Can you work these out from the model? Positions are in its coordinate system, mm. A direction names the side the tool comes from. Give positions to 0.01 mm unless a question says otherwise; leave off trailing zeros. Write each loop counter-clockwise with the first axis right and the second up, starting at its lowest first coordinate (ties: lowest second). Pieces come first, ordered by that corner, then holes.
1. If I drill on probe 1 along X at (y, z) = (21, 17); probe 2 along Y at (x, z) = (34, 2); probe 3 along X at (y, z) = (36, 21), over which ranges is the centre line in solid material (lowest first)?
2. Suppose I cut it at D-D (y = 75). Please give me the cut outline in (x, z), and give its area (3 significant figures).
3. Suppose I cut it at A-A (y = 36.5). Please give me the cut outline in (x, z), and give its area (3 significant figures).
4. Thinking about a two-plate mould opening in Y: for faces 5 (the flat face through (0, -20, 33.02)), 6 (the flat face through (-42.45, -34.32, 12.52)), 7 (the cylindrical face through (16.94, -31.6, 12.88)), which applies, pulls with the +Y half, pulls with the -Y half, needs draft (parallel to the pull), parting line crosses it, or undercut?
5. Suppose I cut it at C-C (z = 18). Please give me the cut outline in (x, y), and give its area (3 significant figures).
6. On a 3-axis mill with a long thin cutter (end or side, diameter ignored), from which of +Z, -Z, +X, -X, +Y, -Y can I reach the whole of each face in a straight line? I mean faces 1 (the flat face through (5.662, 2, 28)), 2 (the cylindrical face through (4.13, -25.59, 27.98)), 3 (the cylindrical face through (4.13, 31.13, 27.98)), 4 (the cylindrical face through (1.708, 21.837, 31.732)). Say none if no direction works.
7. Suppose I cut it at B-B (x = -54.5). Please give me the cut outline in (y, z).
8. I'm going to push flat-ended pins straight in: pin 1 (6 mm diameter, centred on x = 0, y = -11, fed in from +Z); pin 2 (1.1 mm diameter, centred on x = 0, z = 27, fed in from +Y); pin 3 (4 mm diameter, centred on y = 71.5, z = 5, fed in from -X). Where does each tip first touch, or does it pass through?
```python
from build123d import *

# Parameters (mm, degrees)
F1_DEPTH = 25.4
F2_R     = 10.16
F3_R     = 14.427985
F4_DEPTH = 25.401
F6_DEPTH = 5.08
F7_R     = 3.702221
F7_R_2   = 3.8131
F8_DEPTH = 2.54
F9_R     = 5.08


with BuildPart() as f1:
    # F0 (on Top) → F1 (new body)
    with BuildSketch(Plane.XY):
        with BuildLine():
            Line((-0.25744, -76.898574), (75.94256, 0))
            ThreePointArc((75.94256, 0), (-0.25744, 87.97693), (-76.45744, 0))
            Line((-76.45744, 0), (-0.25744, -76.898574))
        make_face()
    extrude(amount=F1_DEPTH)

    # F2
    f2_edges = [f1.edges().sort_by_distance(p)[0] for p in [
        (-0.25744, -76.898574, 12.7),
    ]]
    fillet(f2_edges, radius=F2_R)

    # F3 (on face) → F4 (cut, through all)
    with BuildSketch(Plane.XY.offset(25.4)):
        with Locations((0, 64.553022)):
            Circle(F3_R)
        with Locations((-45.933198, 31.180601)):
            Circle(F3_R)
        with Locations((-28.388277, -22.817112)):
            Circle(F3_R)
        with Locations((28.388277, -22.817112)):
            Circle(F3_R)
        with Locations((45.933198, 31.180601)):
            Circle(F3_R)
    extrude(amount=-F4_DEPTH, mode=Mode.SUBTRACT)

    # F5 (on face) → F6 (join)
    with BuildSketch(Plane.XY.offset(25.4)):
        Polygon((5.661786, 32.575481), (-6.728922, 32.575481), (-5.72427, -27.033882), (5.661786, -27.033882), align=None)
    extrude(amount=F6_DEPTH)

    # F7 (on face) → F8 (join)
    with BuildSketch(Plane.XY.offset(30.48)):
        with Locations((0, 25.121083)):
            Circle(F7_R)
        with Locations((0, -19.945145)):
            Circle(F7_R_2)
    extrude(amount=F8_DEPTH)

    # F9
    f9_edges = [f1.edges().sort_by_distance(p)[0] for p in [
        (-5.72427, -27.033882, 27.94),
        (5.661786, -27.033882, 27.94),
        (5.661786, 32.575481, 27.94),
        (-6.728922, 32.575481, 27.94),
    ]]
    fillet(f9_edges, radius=F9_R)


solid = f1.part
```
Checks:
1. probe 1: x = -76.59 to -56.16, -35.71 to 35.71, 56.16 to 76.08
1. probe 2: y = -42.33 to -36.11, -9.53 to 23.07, 39.29 to 79.94
1. probe 3: x = -73.07 to -59.53, -32.33 to 32.33, 59.53 to 72.55
2. outline: (-43.03, 0) - (-9.95, 0) - (-9.95, 25.4) - (-43.03, 25.4) - close; (9.95, 0) - (42.52, 0) - (42.52, 25.4) - (9.95, 25.4) - close
2. area: 1,670 mm2
3. outline: (-72.9, 0) - (-59.34, 0) - (-59.34, 25.4) - (-72.9, 25.4) - close; (-32.52, 0) - (32.52, 0) - (32.52, 25.4) - (-32.52, 25.4) - close; (59.34, 0) - (72.38, 0) - (72.38, 25.4) - (59.34, 25.4) - close
3. area: 2,330 mm2
4. face 5: needs draft
4. face 6: pulls with the -Y half
4. face 7: undercut
5. outline: (-76.46, 0) - (-7.47, -69.62) arc R10.16 ccw to (6.96, -69.62) - (75.94, 0) arc R76.99 ccw (long way) to start; hole circle Ø28.86 at (-45.93, 31.18); hole circle Ø28.86 at (-28.39, -22.82); hole circle Ø28.86 at (0, 64.55); hole circle Ø28.86 at (28.39, -22.82); hole circle Ø28.86 at (45.93, 31.18)
5. area: 13,600 mm2
6. face 1: +Z, +X, +Y, -Y
6. face 2: +Z, +X, -Y
6. face 3: +Z, +X, +Y
6. face 4: +Z
7. outline: (-22.16, 0) - (19.57, 0) - (19.57, 25.4) - (-22.16, 25.4) - close; (42.79, 0) - (65.62, 0) - (65.62, 25.4) - (42.79, 25.4) - close
8. pin 1: stops at z = 30.48
8. pin 2: stops at y = 32.58
8. pin 3: stops at x = -50.29
